from build123d import *

# Parameters (mm, degrees)
SKETCH1_R           = 1.4
BOSS_EXTRUDE1_DEPTH = 20
SKETCH2_R           = 2.75
BOSS_EXTRUDE2_DEPTH = 1.5
CUT_EXTRUDE1_DEPTH  = 1.3


with BuildPart() as part:
    # Sketch1 → Boss-Extrude1 (new body)
    with BuildSketch(Plane(origin=(0, 0, 0), x_dir=(1, 0, 0), z_dir=(0, 1, 0))):
        with Locations(Location((0, 0, 0), (0, 0, 270))):
            Circle(SKETCH1_R)
    extrude(amount=BOSS_EXTRUDE1_DEPTH)

    # Sketch2 → Boss-Extrude2 (add)
    with BuildSketch(Plane(origin=(0, 20, 0), x_dir=(1, 0, 0), z_dir=(0, 1, 0))):
        with Locations(Location((0, 0, 0), (0, 0, 270))):
            Circle(SKETCH2_R)
    extrude(amount=BOSS_EXTRUDE2_DEPTH)

    # Sketch3 → Cut-Revolve1 (revolve, cut)
    with BuildSketch(Plane(origin=(0, 0, 0), x_dir=(0, 0, -1), z_dir=(1, 0, 0)), mode=Mode.PRIVATE) as cut_revolve1_sk:
        Polygon((1.5, 21.5), (2.75, 20.5), (2.75, 21.5), align=None)
    revolve(cut_revolve1_sk.sketch.rotate(Axis((0, 21.5, 0), (0, -1, 0)), 180), axis=Axis((0, 21.5, 0), (0, -1, 0)), mode=Mode.SUBTRACT)

    # Sketch4 → Cut-Extrude1 (cut)
    with BuildSketch(Plane(origin=(0, 21.5, 0), x_dir=(1, 0, 0), z_dir=(0, 1, 0))):
        Polygon((1.154700538, 0), (0.577350269, 1), (-0.577350269, 1), (-1.154700538, 0), (-0.577350269, -1), (0.577350269, -1), align=None)
    extrude(amount=-CUT_EXTRUDE1_DEPTH, mode=Mode.SUBTRACT)


solid = part.part
Design review of the part built by this model. Coordinates are the model's own, in mm. A direction names the side the tool comes from. Round coordinates to 2 decimals unless told otherwise and drop trailing zeros. Write each loop counter-clockwise with the first axis right and the second up, starting at its lowest first coordinate (ties: lowest second). Pieces come first, ordered by that corner, then holes. Notation, with made-up numbers: (62.25, 3) - (97.25, 3) arc R15 ccw to (97.25, 20) - close; hole circle Ø5 at (71, 0.25). An arc over 180 degrees is marked (long way). Use a Markdown table: item, result. Add a question column.
1. Wall thickness on probe 1 along Z at (x, y) = (0.5, 20.25); probe 2 along Y at (x, z) = (0.15, -0.7); probe 3 along Z at (x, y) = (-0.1, 14.5): over which ranges is each line inside the solid? List them lowest first.
2. For faces 1 (the face through (0, 0, 0)), 2 (the face through (-0.87, 20.86, 0.49)), list the 3-axis set-ups (+Z, -Z, +X, -X, +Y, -Y) from which the entire face can be reached by the end or side of a thin tool; tool diameter is ignored.
3. We need section B-B (y = 8.25). State the section outline as (x, z) points, then the cut area to 3 significant figures.
4. Mouldability with a two-part tool opening along Z and no side actions: class faces 3 (the face through (0.86, 20.86, 0.51)), 4 (the face through (-1.2, 20, 1.2)), 5 (the face through (0.06, 9.86, -1.4)) as +Z half, -Z half, draft (parallel to the pull), parting line (faces both ways), or undercut.
5. We need section A-A (x = 0). State the section outline as (y, z) points, then the cut area to 3 significant figures.
6. Clearance check with flat-ended pins moving along their axes: pin 1 (1.6 mm diameter, centred on x = -0.5, z = 0, fed in from -Y); pin 2 (2 mm diameter, centred on x = 1, y = 17.5, fed in from +Z). State where each tip first meets the part, or that it passes through.
Output:
| question | item | result |
|---|---|---|
| 1 | probe 1 | z = -2.7 to -1, 1 to 2.7 |
| 1 | probe 2 | y = 0 to 20.2 |
| 1 | probe 3 | z = -1.4 to 1.4 |
| 2 | face 1 | +Z, -Z, +X, -X, -Y |
| 2 | face 2 | +Y |
| 3 | outline | circle Ø2.8 at (0, 0) |
| 3 | area | 6.16 mm2 |
| 4 | face 3 | undercut |
| 4 | face 4 | draft |
| 4 | face 5 | parting line |
| 5 | outline | (0, -1.4) - (20, -1.4) - (20, -2.75) - (20.5, -2.75) - (21.5, -1.5) - (21.5, -1) - (20.2, -1) - (20.2, 1) - (21.5, 1) - (21.5, 1.5) - (20.5, 2.75) - (20, 2.75) - (20, 1.4) - (0, 1.4) - close |
| 5 | area | 60.4 mm2 |
| 6 | pin 1 | stops at y = 0 |
| 6 | pin 2 | stops at z = 1.4 |
